Here's how the part is built. I have some questions about the finished solid (model axes, mm). A direction names the side the tool comes from. Round coordinates to 2 decimals unless told otherwise and drop trailing zeros. Loops run counter-clockwise (first coordinate to the right, second up) from the corner with the lowest first, then second, coordinate; pieces in that order, holes last. Notation, with made-up numbers: (-12, 88) - (45, 88) arc R30 cw to (45, 121) - close; hole circle Ø6 at (22, 44.25). An arc over 180 degrees is marked (long way). Answer as a JSON object with one key per item and string values. Group by question number.
1) Which directions (+Z, -Z, +X, -X, +Y, -Y) give clear straight access to the entire face, cutting with the end or side of a thin tool? Please do faces 5 (the face through (0, -1, 600)), 6 (the face through (0, -1, 0)), 7 (the face through (32, -3, 296)), 8 (the face through (-27, -3, 296)), 9 (the face through (10, -10, 296)).
2) I want a section at A-A, the plane z = 550. Please give me the cut outline in (x, y), then the cut area to 3 significant figures.
3) I want a section at D-D, the plane x = -18.5. Please give me the cut outline in (y, z).
4) If I drill on line 1 along X through (y, z) = (-1, 293.5); line 2 along Y through (x, z) = (11.3, 500); line 3 along X through (y, z) = (-12.5, 343.5), over which ranges is the centre line in solid material (lowest first)? Write a range as [from, to].
5) I want a section at C-C, the plane z = 208.5. Please give me the cut outline in (x, y).
6) I want a section at B-B, the plane y = -9.75. Give the number of separate pieces and of enclosed holes in the cut face, then the cut area to 3 significant figures.
7) If we mould it in two halves opening along X, with no side actions, what happens to faces 1 (the face through (1, 0, 296)), 2 (the face through (0, -3, 296)), 3 (the face through (13, -10, 296)), 4 (the face through (-10, -10, 296))? For each: pulls with the +X half, pulls with the -X half, needs draft (parallel to the pull), parting line crosses it, or undercut.
8) Will these pins go through, and if not, where does the flat tip stop? P1, Ø7, axis at y = -9.67, z = 500, coming from the -X side; P2, Ø2, axis at x = 48, z = 125, coming from the -Y side; P3, Ø4, axis at y = -8.5, z = 235, coming from the +X side.
from build123d import *

# Parameters (mm, degrees)
F1_DEPTH = 600
F3_DEPTH = 3.001
F4_R     = 3
F5_DEPTH = 76.001


with BuildPart() as f1:
    # F0 (on Top) → F1 (new body)
    with BuildSketch(Plane.XY):
        Polygon((63, 0), (-63, 0), (-63, -3), (-13, -3), (-13, -16.339283), (-10, -16.339283), (-10, -3), (10, -3), (10, -16.339283), (13, -16.339283), (13, -3), (63, -3), align=None)
    extrude(amount=F1_DEPTH)

    # F2 (on face) → F3 (cut, through all)
    with BuildSketch(Plane.XZ.offset(3)):
        with BuildLine():
            Line((-38, 556), (-48, 556))
            ThreePointArc((-48, 556), (-54, 550), (-48, 544))
            Line((-48, 544), (-38, 544))
            ThreePointArc((-38, 544), (-32, 550), (-38, 556))
        make_face()
        with BuildLine():
            Line((-38, 300), (-48, 300))
            ThreePointArc((-48, 300), (-54, 294), (-48, 288))
            Line((-48, 288), (-38, 288))
            ThreePointArc((-38, 288), (-32, 294), (-38, 300))
        make_face()
        with BuildLine():
            Line((-37.934902, 50), (-47.934902, 50))
            ThreePointArc((-47.934902, 50), (-53.934902, 44), (-47.934902, 38))
            Line((-47.934902, 38), (-37.934902, 38))
            ThreePointArc((-37.934902, 38), (-31.934902, 44), (-37.934902, 50))
        make_face()
        with BuildLine():
            ThreePointArc((47.934902, 38), (53.934902, 44), (47.934902, 50))
            Line((47.934902, 50), (37.934902, 50))
            ThreePointArc((37.934902, 50), (31.934902, 44), (37.934902, 38))
            Line((37.934902, 38), (47.934902, 38))
        make_face()
        with BuildLine():
            ThreePointArc((48, 288), (54, 294), (48, 300))
            Line((48, 300), (38, 300))
            ThreePointArc((38, 300), (32, 294), (38, 288))
            Line((38, 288), (48, 288))
        make_face()
        with BuildLine():
            ThreePointArc((38, 556), (32, 550), (38, 544))
            Line((38, 544), (48, 544))
            ThreePointArc((48, 544), (54, 550), (48, 556))
            Line((48, 556), (38, 556))
        make_face()
    extrude(amount=-F3_DEPTH, mode=Mode.SUBTRACT)

    # F4 (on face) → F5 (cut, through all)
    with BuildSketch(Plane(origin=(-13, 0, 0), x_dir=(0, -1, 0), z_dir=(-1, 0, 0))):
        with Locations((9.669641, 500)):
            Circle(F4_R)
        with Locations((9.669641, 300)):
            Circle(F4_R)
        with Locations((9.669641, 100)):
            Circle(F4_R)
    extrude(amount=-F5_DEPTH, mode=Mode.SUBTRACT)


solid = f1.part
Outcome:
{
 "1": {"face 5": "+Z, +X, -X, +Y, -Y", "face 6": "-Z, +X, -X, +Y, -Y", "face 7": "+Z, -Z, +X, -Y", "face 8": "+Z, -Z, -X, -Y", "face 9": "+Z, -Z, -Y"},
 "2": {"outline": "(-63, -3) - (-54, -3) - (-54, 0) - (-63, 0) - close; (-32, -3) - (-13, -3) - (-13, -16.34) - (-10, -16.34) - (-10, -3) - (10, -3) - (10, -16.34) - (13, -16.34) - (13, -3) - (32, -3) - (32, 0) - (-32, 0) - close; (54, -3) - (63, -3) - (63, 0) - (54, 0) - close", "area": "326 mm^2"},
 "3": {"outline": "(-3, 0) - (0, 0) - (0, 600) - (-3, 600) - close"},
 "4": {"line 1": "[-63, -53.98], [-32.02, 32.02], [53.98, 63]", "line 2": "[-16.34, -12.67], [-6.67, 0]", "line 3": "[-13, -10], [10, 13]"},
 "5": {"outline": "(-63, -3) - (-13, -3) - (-13, -16.34) - (-10, -16.34) - (-10, -3) - (10, -3) - (10, -16.34) - (13, -16.34) - (13, -3) - (63, -3) - (63, 0) - (-63, 0) - close"},
 "6": {"separate pieces": "8", "enclosed holes": "0", "area": "3,490 mm^2"},
 "7": {"face 1": "needs draft", "face 2": "undercut", "face 3": "pulls with the +X half", "face 4": "undercut"},
 "8": {"P1": "x = -13", "P2": "y = -3", "P3": "x = 13"}
}
